from build123d import *

# Parameters (mm, degrees)
BOSS_EXTRUDE1_DEPTH       = 20.32
TAP_DRILL_FOR_2_56_TAP1_D = 1.778


with BuildPart() as part:
    # Sketch1 → Boss-Extrude1 (new body)
    with BuildSketch(Plane(origin=(0, 0, 0), x_dir=(1, 0, 0), z_dir=(0, 1, 0))):
        with BuildLine():
            Line((0, 13.208), (0, 9.398))
            ThreePointArc((0, 9.398), (9.398, 0), (0, -9.398))
            Line((0, -9.398), (0, -13.208))
            ThreePointArc((0, -13.208), (13.208, 0), (0, 13.208))
        make_face()
    extrude(amount=BOSS_EXTRUDE1_DEPTH)

    # Tap Drill for #2-56 Tap1 (through all)
    with Locations(Plane(origin=(0, 15.24, -11.303), x_dir=(0, 0, -1), z_dir=(-1, 0, 0))):
        with Locations((0, 0), (-22.606, 0), (-22.606, 10.16), (0, 10.16)):
            Hole(TAP_DRILL_FOR_2_56_TAP1_D / 2)


solid = part.part
Verification items for the finished model (mm, model axes). Give positions to 0.01 mm unless a question says otherwise; leave off trailing zeros. Write each loop counter-clockwise with the first axis right and the second up, starting at its lowest first coordinate (ties: lowest second). Pieces come first, ordered by that corner, then holes. Notation, with made-up numbers: M 5.5,0 L 16.5,0 A25 ccw 16.5,38 Z; hole C 55,52 d10. An arc over 180 degrees is marked long. Use CSV: the item, a comma, the result in double quotes.
1) Material ranges on line 1 along Y through (x, z) = (1.25, 11); line 2 along Z through (x, y) = (1.5, 5.25); line 3 along Z through (x, y) = (3.75, 15.24), recorded low to high.
Final values:
line 1,"0 to 4.24, 5.92 to 14.4, 16.08 to 20.32"
line 2,"-13.12 to -12.18, -10.43 to -9.28, 9.28 to 10.43, 12.18 to 13.12"
line 3,"-12.66 to -12.19, -10.41 to -8.62, 8.62 to 10.41, 12.19 to 12.66"
2) Go/stop test with flat-tipped pins: pin 1 Ø2 at (y, z) = (13, -7.5) entering from -X; pin 2 Ø3 at (y, z) = (15.24, 11.303) entering from +X; pin 3 Ø2 at (y, z) = (10.5, 1) entering from -X. Record where each tip stops, or that it passes through.
Final values:
pin 1,"x = 4.01"
pin 2,"x = 8.85"
pin 3,"x = 9.18"
3) Cross-section at B-B (x = 2). Enter the section's corners in (y, z).
Final values:
outline,"M 0,-13.06 L 20.32,-13.06 L 20.32,-9.18 L 0,-9.18 Z; M 0,9.18 L 20.32,9.18 L 20.32,13.06 L 0,13.06 Z; hole C 5.08,-11.3 d1.78; hole C 5.08,11.3 d1.78; hole C 15.24,-11.3 d1.78; hole C 15.24,11.3 d1.78"
4) Cross-section at C-C (y = 12). Enter the section's corners in (x, z), plus the area to 3 significant figures.
Final values:
outline,"M 0,-13.21 A13.21 ccw 0,13.21 L 0,9.4 A9.4 cw 0,-9.4 Z"
area,"135 mm²"
5) Release check for a two-part mould opening along Z. For faces 1 (the face through (13.205, 10.018, 0.29)), 2 (the face through (3.216, 15.201, 10.415)), 3 (the face through (0, 10, -11)), 4 (the face through (3.216, 4.813, -10.455)) record: released by +Z, released by -Z, zero draft, split by the parting line, or undercut.
Final values:
face 1,"split by the parting line"
face 2,"undercut"
face 3,"zero draft"
face 4,"undercut"
6) Cross-section at D-D (z = -6.5). Enter the section's corners in (x, y).
Final values:
outline,"M 6.79,0 L 11.5,0 L 11.5,20.32 L 6.79,20.32 Z"
7) Cross-section at A-A (y = 5.08). Enter the section's corners in (x, z).
Final values:
outline,"M 0,-13.21 A13.21 ccw 5.08,-12.19 L 0,-12.19 Z; M 0,-10.41 L 8.12,-10.41 A13.21 ccw 8.12,10.41 L 0,10.41 L 0,9.4 A9.4 cw 0,-9.4 Z; M 0,12.19 L 5.08,12.19 A13.21 ccw 0,13.21 Z"
